```python
from build123d import *

# Parameters (mm, degrees)
RESSALTO_EXTRUS_O1_DEPTH   = 10
CORTE_EXTRUS_O1_DEPTH      = 2
CORTE_EXTRUS_O1_DEPTH_BACK = 2.6
ESBO_O3_R                  = 1.7
CORTE_EXTRUS_O2_DEPTH      = 1.9
FILETE2_R                  = 3


with BuildPart() as part:
    # Esboço1 → Ressalto-extrusão1 (new body)
    with BuildSketch(Plane.XY):
        with BuildLine():
            Line((3.2, -5.25), (8.7, -5.25))
            Line((8.7, -5.25), (8.7, 8.75))
            Line((8.7, 8.75), (-8.7, 8.75))
            Line((-8.7, 8.75), (-8.7, -5.25))
            Line((-8.7, -5.25), (-3.2, -5.25))
            ThreePointArc((-3.2, -5.25), (-5.321320344, -4.371320344), (-6.2, -2.25))
            Line((-6.2, -2.25), (-6.2, 2.25))
            ThreePointArc((-6.2, 2.25), (-5.321320344, 4.371320344), (-3.2, 5.25))
            Line((-3.2, 5.25), (3.2, 5.25))
            ThreePointArc((3.2, 5.25), (5.321320344, 4.371320344), (6.2, 2.25))
            Line((6.2, 2.25), (6.2, -2.25))
            ThreePointArc((6.2, -2.25), (5.321320344, -4.371320344), (3.2, -5.25))
        make_face()
    extrude(amount=RESSALTO_EXTRUS_O1_DEPTH)

    # Esboço2 → Corte-extrusão1 (cut, two sides)
    with BuildSketch(Plane.XZ.offset(-5.25)) as corte_extrus_o1_sk:
        Polygon((1.616580754, 2.2), (3.233161507, 5), (1.616580754, 7.8), (-1.616580754, 7.8), (-3.233161507, 5), (-1.616580754, 2.2), align=None)
    extrude(amount=CORTE_EXTRUS_O1_DEPTH, mode=Mode.SUBTRACT)
    extrude(corte_extrus_o1_sk.sketch, amount=-CORTE_EXTRUS_O1_DEPTH_BACK, mode=Mode.SUBTRACT)

    # Esboço3 → Corte-extrusão2 (cut, through all)
    with BuildSketch(Plane.XZ.offset(-7.85)):
        with Locations((0, 5)):
            Circle(ESBO_O3_R)
    extrude(amount=-CORTE_EXTRUS_O2_DEPTH, mode=Mode.SUBTRACT)

    # Filete2
    filete2_edges = [part.edges().sort_by_distance(p)[0] for p in [
        (-8.7, 8.75, 5),
        (8.7, 8.75, 5),
    ]]
    fillet(filete2_edges, radius=FILETE2_R)


solid = part.part
```
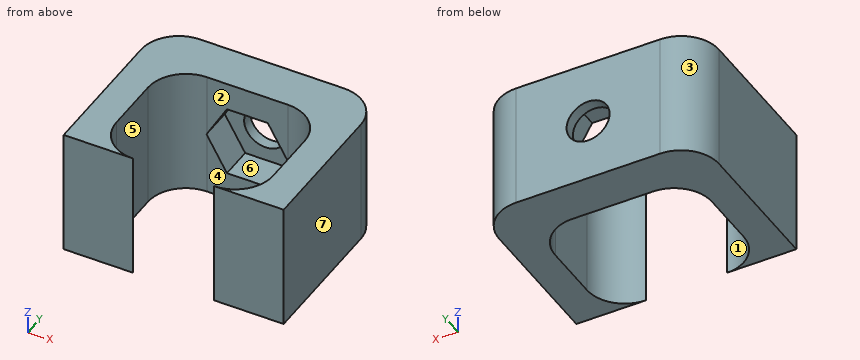
Source: CAD feature listing. Evaluate the final solid. Frame: model axes, mm. Face numbers are marked on the shaded views. A direction names the side the tool comes from. Coordinates: 2 decimals unless noted, no trailing zeros. Loops run counter-clockwise (first coordinate to the right, second up) from the corner with the lowest first, then second, coordinate; pieces in that order, holes last. Notation, with made-up numbers: (-36.5, 24.25) - (19.5, 24.25) arc R21 ccw to (19.5, 56.25) - close; hole circle Ø1 at (58.5, -34.75). An arc over 180 degrees is marked (long way). Answer as CSV lines item,"result".
1. Section B-B (y = -4). Return loops of the section in (x, z), then the cut area to 3 significant figures.
Established:
outline,"(-8.7, 0) - (-5.64, 0) - (-5.64, 10) - (-8.7, 10) - close; (5.64, 0) - (8.7, 0) - (8.7, 10) - (5.64, 10) - close"
area,"61.3 mm2"
2. Mould query, pull axis Y, two halves, no side actions, for the marked faces 1, 2 and 3. Classes: released by +Y, released by -Y, zero draft, split by the parting line, or undercut.
Established:
face 1,"undercut"
face 2,"released by -Y"
face 3,"released by +Y"
3. Ray query, line 1 (Z direction, x = 0, y = 8.25); line 2 (Z direction, x = -0.75, y = 6.25); line 3 (X direction, y = -1.5, z = 6.25). Return the intervals inside material, ascending.
Established:
line 1,"z = 0 to 3.3, 6.7 to 10"
line 2,"z = 0 to 2.2, 7.8 to 10"
line 3,"x = -8.7 to -6.2, 6.2 to 8.7"
4. Section D-D (x = 5.5). Return loops of the section in (y, z).
Established:
outline,"(-5.25, 0) - (-4.18, 0) - (-4.18, 10) - (-5.25, 10) - close; (4.18, 0) - (8.75, 0) - (8.75, 10) - (4.18, 10) - close"
5. Contact query for a flat-ended pin moving along its axis: pin 1 (6 mm diameter, centred on x = 0, z = 4, fed in from -Y). Output: stop coordinate, or through.
Established:
pin 1,"stops at y = 5.25"
6. Section C-C (z = 6). Return loops of the section in (x, y).
Established:
outline,"(-8.7, -5.25) - (-3.2, -5.25) arc R3 cw to (-6.2, -2.25) - (-6.2, 2.25) arc R3 cw to (-3.2, 5.25) - (-2.66, 5.25) - (-2.66, 7.85) - (-1.37, 7.85) - (-1.37, 8.75) - (-5.7, 8.75) arc R3 ccw to (-8.7, 5.75) - close; (1.37, 7.85) - (2.66, 7.85) - (2.66, 5.25) - (3.2, 5.25) arc R3 cw to (6.2, 2.25) - (6.2, -2.25) arc R3 cw to (3.2, -5.25) - (8.7, -5.25) - (8.7, 5.75) arc R3 ccw to (5.7, 8.75) - (1.37, 8.75) - close"
7. Section A-A (x = 0). Return loops of the section in (y, z), then the cut area to 3 significant figures.
Established:
outline,"(5.25, 0) - (8.75, 0) - (8.75, 3.3) - (7.85, 3.3) - (7.85, 2.2) - (5.25, 2.2) - close; (5.25, 7.8) - (7.85, 7.8) - (7.85, 6.7) - (8.75, 6.7) - (8.75, 10) - (5.25, 10) - close"
area,"17.4 mm2"
8. Reachability of the marked faces 4, 5, 6 and 7 from +Z, -Z, +X, -X, +Y, -Y: full face, straight path, thin tool, end or side. Return the list, or none.
Established:
face 4,"+Z, -Z, -Y"
face 5,"+Z, -Z"
face 6,"-Y"
face 7,"+Z, -Z, +X, +Y, -Y"
